For this review, take the finished solid that the model builds, in its own axes (mm). Face numbers are marked on the shaded views. A direction names the side the tool comes from. Coordinates: 2 decimals unless noted, no trailing zeros. Order: outer loops, then holes, each group sorted by start corner. A loop starts at its lowest first (then second) coordinate and runs counter-clockwise, first axis right, second up. Notation, with made-up numbers: (-20, 79) -> (-6, 79) arc R23 cw to (-6, 102) -> close; hole circle Ø7 at (24.5, 28.5). An arc over 180 degrees is marked (long way). Write item = value, one per line. Start each with the question number.
1) Draft analysis for pull direction X (two halves, no side actions). For the marked faces 1, 2, 3 and 4, state which applies: +X half, -X half, draft (parallel to the pull), parting line (faces both ways), or undercut.
2) Wall thickness on probe 1 along Y at (x, z) = (53, 2.8); probe 2 along Y at (x, z) = (53.75, 5.75); probe 3 along X at (y, z) = (26.25, 5.3): over which ranges is each line inside the solid? List them lowest first. Write a range as [from, to].
3) Insertion check: pin 1 Ø1 at (y, z) = (18, 1.5) entering from +X; pin 2 Ø1.5 at (y, z) = (22.5, 1) entering from -X; pin 3 Ø5.5 at (x, y) = (52.95, 25.42) entering from +Z; pin 4 Ø1.2 at (x, z) = (49, 1.5) entering from -Y. Each pin has a flat end and moves straight along its axis. Give the tip position at first contact, or say it passes through.
4) Consider section B-B on x = 53. Give the boundary of the cut face in (y, z), and give its area (3 significant figures).
5) Consider section A-A on y = 28. Give the boundary of the cut face in (x, z).
6) Consider section C-C on z = 1.3. Give the boundary of the cut face in (x, y), and give its area (3 significant figures).
7) Consider section D-D on y = 15.5. Give the boundary of the cut face in (x, z), and give its area (3 significant figures).
8) Machinability: for the marked faces 5, 6 and 7, which of the approach directions +Z, -Z, +X, -X, +Y, -Y give a long, thin tool a straight path to every point of the face, cutting with its end or side? Answer none if there is none.
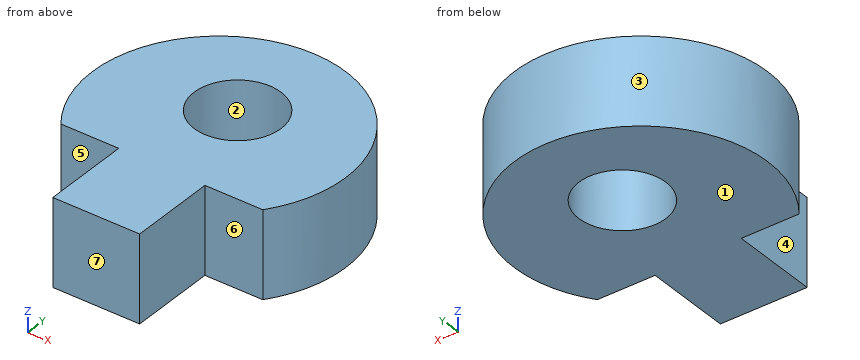
from build123d import *

# Parameters (mm, degrees)
MODEL_R             = 3
BOSS_EXTRUDE1_DEPTH = 6


with BuildPart() as part:
    # Model → Boss-Extrude1 (new body)
    with BuildSketch(Plane.XY):
        with BuildLine():
            Line((55.946512191, 18.417561913), (55.946512191, 12.417561913))
            Line((55.946512191, 12.417561913), (49.946512191, 12.417561913))
            Line((49.946512191, 12.417561913), (49.946512191, 18.479362937))
            Line((49.946512191, 18.479362937), (45.946512191, 18.479362937))
            ThreePointArc((45.946512191, 18.479362937), (53.008176567, 32.417507278), (59.946512191, 18.417561913))
            Line((59.946512191, 18.417561913), (55.946512191, 18.417561913))
        make_face()
        with Locations((52.946512191, 25.417561913)):
            Circle(MODEL_R, mode=Mode.SUBTRACT)
    extrude(amount=BOSS_EXTRUDE1_DEPTH)


solid = part.part
Answer sheet:
q1.face_1 = draft
q1.face_2 = undercut
q1.face_3 = parting line
q1.face_4 = -X half
q2.probe_1 = [12.42, 22.42], [28.42, 32.42]
q2.probe_2 = [12.42, 22.53], [28.31, 32.38]
q2.probe_3 = [44.62, 50.06], [55.83, 61.32]
q3.pin_1 = 60.01
q3.pin_2 = 44.24
q3.pin_3 = through
q3.pin_4 = 18.48
q4.outline = (12.42, 0) -> (22.42, 0) -> (22.42, 6) -> (12.42, 6) -> close; (28.42, 0) -> (32.42, 0) -> (32.42, 6) -> (28.42, 6) -> close
q4.area = 84.0 mm2
q5.outline = (45.37, 0) -> (51.42, 0) -> (51.42, 6) -> (45.37, 6) -> close; (54.47, 0) -> (60.57, 0) -> (60.57, 6) -> (54.47, 6) -> close
q6.outline = (45.95, 18.48) -> (49.95, 18.48) -> (49.95, 12.42) -> (55.95, 12.42) -> (55.95, 18.42) -> (59.95, 18.42) arc R8.74 ccw (long way) to start; hole circle Ø6 at (52.95, 25.42)
q6.area = 213 mm2
q7.outline = (49.95, 0) -> (55.95, 0) -> (55.95, 6) -> (49.95, 6) -> close
q7.area = 36.0 mm2
q8.face_5 = +Z, -Z, -X, -Y
q8.face_6 = +Z, -Z, +X, -Y
q8.face_7 = +Z, -Z, +X, -X, -Y
